Geometry check sheet. Reference: drawing and pictorial views, mm from the part's lowest x, y, z. A direction names the side the tool comes from. Give positions to 0.01 mm unless a question says otherwise; leave off trailing zeros. Order: outer loops, then holes, each group sorted by start corner. A loop starts at its lowest first (then second) coordinate and runs counter-clockwise, first axis right, second up.
Item 1: Sectioned sample at A-A on z = 8.5. Record the boundary of the cut face in (x, y), and give its area (3 significant figures).
Item 2: Access from +Z, -Z, +X, -X, +Y, -Y to the whole of each face (thin tool, end or side, straight path). Record for the marked faces 1 and 2.
Item 3: Gauge pin test, flat ends, axial feed: P1, Ø1, axis at x = 10.5, z = 8, coming from the +Y side; P2, Ø1, axis at y = 10, z = 6, coming from the +X side; P3, Ø5, axis at y = 9, z = 24.5, coming from the -X side; P4, Ø2, axis at x = 8.5, y = 10, coming from the +Z side. Record the tip position at first contact, or that the pin passes through.
Item 4: Material ranges on line 1 along Y through (x, z) = (6.75, 16); line 2 along Z through (x, y) = (4, 8.25); line 3 along Y through (x, z) = (2, 29), recorded low to high.
Item 5: Sectioned sample at B-B on z = 26. Record the boundary of the cut face in (x, y).
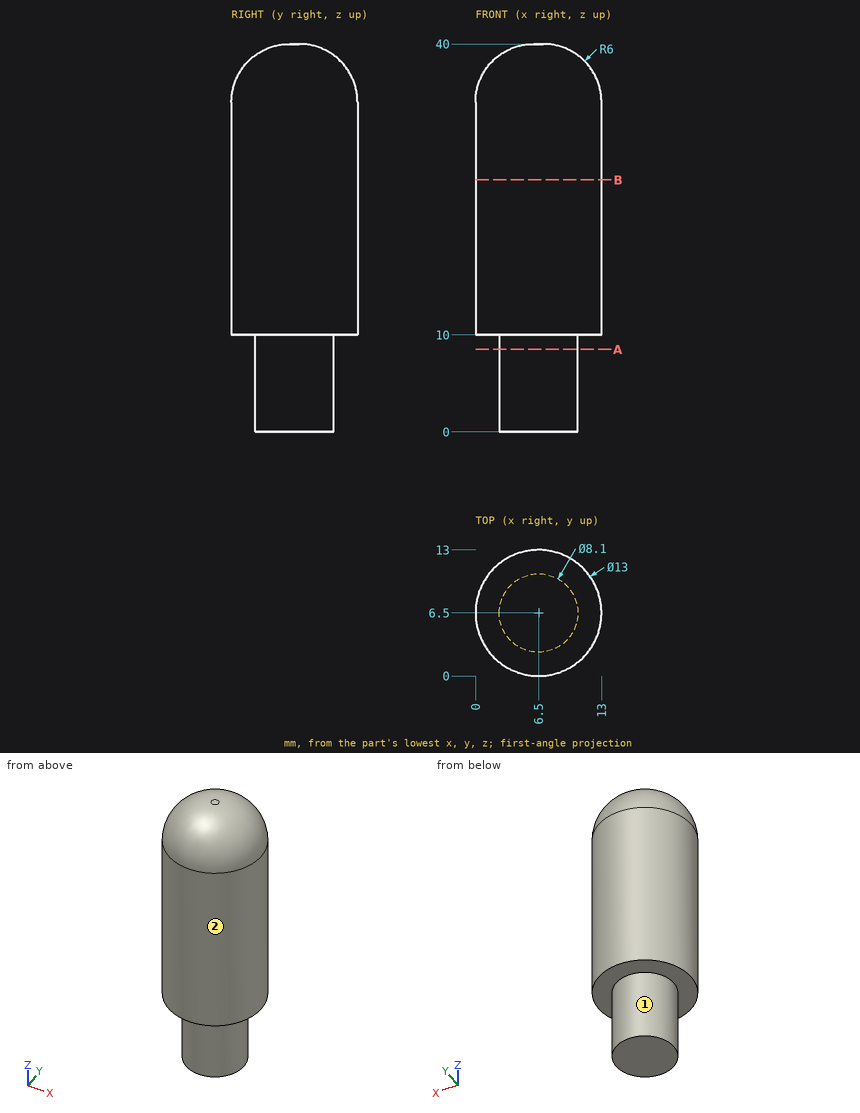
Report:
1. outline: circle Ø8.1 at (6.5, 6.5)
1. area: 51.5 mm2
2. face 1: -Z
2. face 2: +Z, -Z
3. P1: stops at y = 8.54
3. P2: stops at x = 9.22
3. P3: stops at x = 0
3. P4: stops at z = 39.44
4. line 1: y = 0 to 13
4. line 2: z = 0 to 39.43
4. line 3: y = 1.81 to 11.19
5. outline: circle Ø13 at (6.5, 6.5)
